Design review of the part built by this model. Coordinates are the model's own, in mm. Face numbers are marked on the shaded views. Give positions to 0.01 mm unless a question says otherwise; leave off trailing zeros. Loops run counter-clockwise (first coordinate to the right, second up) from the corner with the lowest first, then second, coordinate; pieces in that order, holes last.
from build123d import *
from OCP.BRepAlgoAPI import BRepAlgoAPI_Cut
from OCP.TopTools import TopTools_ListOfShape

# Parameters (mm, degrees)
SKETCH3_R           = 14.605
SKETCH3_R_2         = 12.7
BOSS_EXTRUDE2_DEPTH = 80.01
SKETCH4_R           = 14.605
BOSS_EXTRUDE3_DEPTH = 40.005
SKETCH5_R           = 12.7
CUT_EXTRUDE1_DEPTH  = 40.005
SKETCH6_R           = 14.605
BOSS_EXTRUDE4_DEPTH = 40.005
SKETCH7_R           = 12.7
CUT_EXTRUDE2_DEPTH  = 40.005
SKETCH8_R           = 12.7
CUT_EXTRUDE3_DEPTH  = 98.991837283
CUT_EXTRUDE4_REACH  = 106.806
SKETCH9_R           = 12.7


with BuildPart() as part:
    # Sketch3 → Boss-Extrude2 (new body)
    with BuildSketch(Plane(origin=(0, 0, 0), x_dir=(1, 0, 0), z_dir=(0, 1, 0))):
        with Locations(Location((0, 0, 0), (0, 0, 270))):
            Circle(SKETCH3_R)
        with Locations(Location((0, 0, 0), (0, 0, 270))):
            Circle(SKETCH3_R_2, mode=Mode.SUBTRACT)
    extrude(amount=BOSS_EXTRUDE2_DEPTH)

    # Sketch4 → Boss-Extrude3 (add)
    with BuildSketch(Plane.XY):
        with Locations((0, 40.005)):
            Circle(SKETCH4_R)
    extrude(amount=BOSS_EXTRUDE3_DEPTH)

    # Sketch5 → Cut-Extrude1 (cut)
    with BuildSketch(Plane.XY.offset(40.005)):
        with Locations((0, 40.005)):
            Circle(SKETCH5_R)
    extrude(amount=-CUT_EXTRUDE1_DEPTH, mode=Mode.SUBTRACT)

    # Sketch6 → Boss-Extrude4 (add)
    with BuildSketch(Plane(origin=(0, 0, 0), x_dir=(0, 0, -1), z_dir=(1, 0, 0))):
        with Locations((0, 40.005)):
            Circle(SKETCH6_R)
    extrude(amount=BOSS_EXTRUDE4_DEPTH)

    # Sketch7 → Cut-Extrude2 (cut)
    with BuildSketch(Plane(origin=(40.005, 0, 0), x_dir=(0, 0, -1), z_dir=(1, 0, 0))):
        with Locations((0, 40.005)):
            Circle(SKETCH7_R)
    extrude(amount=-CUT_EXTRUDE2_DEPTH, mode=Mode.SUBTRACT)


with BuildPart() as cut_extrude3_tool:
    # Sketch8 → Cut-Extrude3 (new, through all)
    with BuildSketch(Plane(origin=(0, 80.01, 0), x_dir=(1, 0, 0), z_dir=(0, 1, 0))):
        with Locations(Location((0, 0, 0), (0, 0, 270))):
            Circle(SKETCH8_R)
    extrude(amount=-CUT_EXTRUDE3_DEPTH)


with BuildPart() as part_1:
    add(part.part)

    # Cut-Extrude3: cut by cut_extrude3_tool, with a tolerance
    cut_extrude3_stock = TopTools_ListOfShape()
    cut_extrude3_stock.Append(part_1.part.wrapped)
    cut_extrude3_tools = TopTools_ListOfShape()
    cut_extrude3_tools.Append(cut_extrude3_tool.part.wrapped)
    cut_extrude3_cut = BRepAlgoAPI_Cut()
    cut_extrude3_cut.SetArguments(cut_extrude3_stock)
    cut_extrude3_cut.SetTools(cut_extrude3_tools)
    cut_extrude3_cut.SetFuzzyValue(0.00001)
    cut_extrude3_cut.Build()
    add(Compound.cast(cut_extrude3_cut.Shape()).solids(), mode=Mode.REPLACE)

    # Sketch9 → Cut-Extrude4 (cut, up to next)
    with BuildSketch(Plane.XY.offset(40.005), mode=Mode.PRIVATE) as cut_extrude4_sk1:
        with Locations((0, 40.005)):
            Circle(SKETCH9_R)
    cut_extrude4_tool1 = extrude(cut_extrude4_sk1.sketch, amount=-CUT_EXTRUDE4_REACH, mode=Mode.PRIVATE) & part_1.part
    add(cut_extrude4_tool1.solids().sort_by_distance((0, 40.005, 40.005))[0], mode=Mode.SUBTRACT)


solid = part_1.part
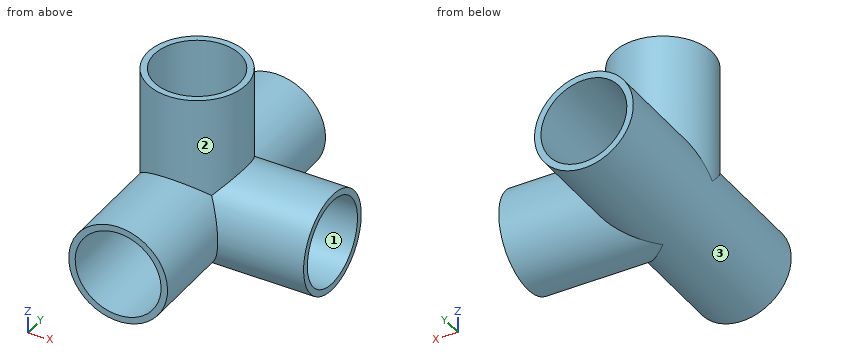
Q1. Take a section at A-A (z = 33.5). Give the boundary of the cut face in (x, y) (3 decimals).
Results:
outline: circle Ø29.21 at (0, 40.005); hole circle Ø25.4 at (0, 40.005)
Q2. Take a section at C-C (x = 36.5). Give the boundary of the cut face in (y, z) (3 decimals).
Results:
outline: circle Ø29.21 at (40.005, 0); hole circle Ø25.4 at (40.005, 0)
Q3. Draft analysis for pull direction Z (two halves, no side actions). For the marked faces 1, 2 and 3, state which applies: pulls with the +Z half, pulls with the -Z half, needs draft (parallel to the pull), parting line crosses it, or undercut.
Results:
face 1: undercut
face 2: needs draft
face 3: parting line crosses it
Q4. Take a section at B-B (z = -4.5). Give the boundary of the cut face in (x, y) (3 decimals), plus the area to 3 significant figures.
Results:
outline: (-13.894, 0) - (-11.876, 0) - (-11.876, 80.01) - (-13.894, 80.01) - close; (11.876, 0) - (13.894, 0) - (13.894, 26.111) - (40.005, 26.111) - (40.005, 28.129) - (11.876, 28.129) - close; (11.876, 51.881) - (40.005, 51.881) - (40.005, 53.899) - (13.894, 53.899) - (13.894, 80.01) - (11.876, 80.01) - close
area: 380 mm2
Q5. Insertion check: pin 1 (1 mm diameter, centred on y = 64, z = -6, fed in from +X); pin 2 (4 mm diameter, centred on y = 20, z = -8.5, fed in from +X); pin 3 (4 mm diameter, centred on x = 6, y = 16.5, fed in from +Z). Each pin has a flat end and moves straight along its axis. Give the tip position at first contact, or say it passes through.
Results:
pin 1: stops at x = 13.53
pin 2: stops at x = 13.08
pin 3: stops at z = 14.05
Q6. Wall thickness on line 1 (Z direction, x = 0, y = 21) (3 decimals); line 2 (Y direction, x = 0, z = 27.5) (3 decimals); line 3 (Z direction, x = -3, y = 18): over which ranges is each line inside the solid? List them lowest first.
Results:
line 1: z = -14.605 to -12.7, 12.7 to 14.605
line 2: y = 25.4 to 27.305, 52.705 to 54.61
line 3: z = -14.29 to -12.34, 12.34 to 14.29
